```python
from build123d import *

# Parameters (mm, degrees)
SKETCH051_R             = 1.5
PAD022_DEPTH            = 3.5
SKETCH052_R             = 17.5
PAD003_DEPTH            = 12.5
SKETCH053_R             = 18.25
PAD004_DEPTH            = 4
SKETCH005_R             = 8
PAD023_DEPTH            = 2
SKETCH006_R             = 2.5
PAD021_DEPTH            = 12
BODY024_PLACEMENT_ANGLE = 90


with BuildPart() as part:
    # Sketch051 → Pad022 (new body)
    with BuildSketch(Plane.XY):
        with BuildLine():
            ThreePointArc((-16.780137, -7.175619), (0.077574, -18.249835), (16.840532, -7.032709))
            Line((23.588818, -4.651296), (16.840532, -7.032709))
            ThreePointArc((23.588818, -4.651296), (26.754582, -0.217457), (23.665308, 4.270011))
            Line((16.947438, 6.77103), (23.665308, 4.270011))
            ThreePointArc((16.947438, 6.77103), (0.049146, 18.249934), (-16.910725, 6.862207))
            Line((-16.910725, 6.862207), (-23.684267, 4.419805))
            ThreePointArc((-23.684267, 4.419805), (-26.870918, -0.10661), (-23.703302, -4.646365))
            Line((-23.703302, -4.646365), (-16.780137, -7.175619))
        make_face()
        with Locations((-22.015205, 0)):
            Circle(SKETCH051_R, mode=Mode.SUBTRACT)
        with Locations((21.805187, 0)):
            Circle(SKETCH051_R, mode=Mode.SUBTRACT)
    extrude(amount=PAD022_DEPTH)

    # Sketch052 (on Face11 of Pad022) → Pad003 (join)
    with BuildSketch(Plane(origin=(0, 0, 0), x_dir=(1, 0, 0), z_dir=(0, 0, -1))):
        Circle(SKETCH052_R)
    extrude(amount=PAD003_DEPTH)

    # Sketch053 (on Face14 of Pad003) → Pad004 (join)
    with BuildSketch(Plane(origin=(0, 0, -12.5), x_dir=(1, 0, 0), z_dir=(0, 0, -1))):
        Circle(SKETCH053_R)
    extrude(amount=PAD004_DEPTH)

    # Sketch005 (on Face16 of Pad004) → Pad023 (join)
    with BuildSketch(Plane.XY.offset(3.5)):
        Circle(SKETCH005_R)
    extrude(amount=PAD023_DEPTH)

    # Sketch006 (on Face18 of Pad023) → Pad021 (join)
    with BuildSketch(Plane.XY.offset(5.5)):
        Circle(SKETCH006_R)
    extrude(amount=PAD021_DEPTH)


with BuildPart() as part_1:
    # Body024 placement: moved
    add(part.part.moved(Location((0, 9.5, 80.3))).rotate(Axis((0, 9.5, 80.3), (-1, 0, 0)), BODY024_PLACEMENT_ANGLE))


solid = part_1.part
```
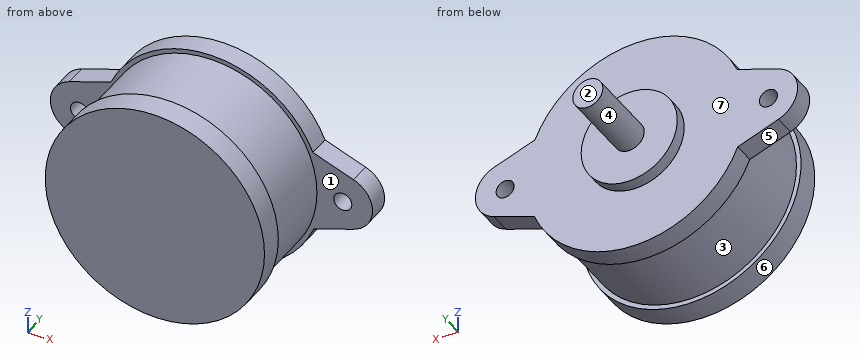
Geometry check sheet. Reference: the model listing, model coordinates, mm. Face numbers are marked on the shaded views. A direction names the side the tool comes from. Coordinates: 2 decimals unless noted, no trailing zeros. Loops run counter-clockwise (first coordinate to the right, second up) from the corner with the lowest first, then second, coordinate; pieces in that order, holes last.
Item 1: Sectioned sample at C-C, the plane y = 25.5. Record the boundary of the cut face in (x, z).
Item 2: Access from +Z, -Z, +X, -X, +Y, -Y to the whole of each face (thin tool, end or side, straight path). Record for the marked faces 5, 6 and 7.
Item 3: Release check for a two-part mould opening along Y. For the marked faces 1, 2, 3 and 4 record: released by +Y, released by -Y, zero draft, split by the parting line, or undercut.
Item 4: Sectioned sample at A-A, the plane z = 80.3. Record the boundary of the cut face in (x, y), then the cut area to 3 significant figures.
Item 5: Thickness scan on line 1 (X direction, y = 10.35, z = 80.3); line 2 (Y direction, x = 16, z = 87.5); line 3 (X direction, y = 10, z = 80). Record the ranges inside material, lowest first.
Item 6: Sectioned sample at D-D, the plane z = 89.5. Record the boundary of the cut face in (x, y), then the cut area to 3 significant figures.
Item 7: Go/stop test with flat-tipped pins: pin 1 Ø4 at (x, z) = (11.5, 81) entering from +Y; pin 2 Ø10 at (x, y) = (-13.5, 6) entering from -Z; pin 3 Ø11 at (x, z) = (9, 74.5) entering from +Y. Record where each tip stops, or that it passes through.
Item 8: Sectioned sample at B-B, the plane x = 0. Record the boundary of the cut face in (y, z).
Check result:
1. outline: circle Ø5 at (0, 80.3)
2. face 5: -Z, -X, +Y, -Y
2. face 6: -Y
2. face 7: +Y
3. face 1: undercut
3. face 2: released by +Y
3. face 3: undercut
3. face 4: zero draft
4. outline: (-26.87, 9.5) - (-23.52, 9.5) - (-23.52, 13) - (-26.87, 13) - close; (-20.52, 9.5) - (-17.5, 9.5) - (-17.5, -3) - (-18.25, -3) - (-18.25, -7) - (18.25, -7) - (18.25, -3) - (17.5, -3) - (17.5, 9.5) - (20.31, 9.5) - (20.31, 13) - (8, 13) - (8, 15) - (2.5, 15) - (2.5, 27) - (-2.5, 27) - (-2.5, 15) - (-8, 15) - (-8, 13) - (-20.52, 13) - close; (23.31, 9.5) - (26.75, 9.5) - (26.75, 13) - (23.31, 13) - close
4. area: 842 mm2
5. line 1: x = -26.87 to -23.52, -20.52 to 20.31, 23.31 to 26.75
5. line 2: y = -7 to -3, 9.5 to 13
5. line 3: x = -26.85 to -23.48, -20.55 to 20.34, 23.27 to 26.73
6. outline: (-15.76, -7) - (15.76, -7) - (15.76, -3) - (14.89, -3) - (14.89, 9.5) - (15.76, 9.5) - (15.76, 13) - (-15.76, 13) - (-15.76, 9.5) - (-14.89, 9.5) - (-14.89, -3) - (-15.76, -3) - close
6. area: 609 mm2
7. pin 1: stops at y = 13
7. pin 2: stops at z = 64.99
7. pin 3: stops at y = 15
8. outline: (-7, 62.05) - (-3, 62.05) - (-3, 62.8) - (9.5, 62.8) - (9.5, 62.05) - (13, 62.05) - (13, 72.3) - (15, 72.3) - (15, 77.8) - (27, 77.8) - (27, 82.8) - (15, 82.8) - (15, 88.3) - (13, 88.3) - (13, 98.55) - (9.5, 98.55) - (9.5, 97.8) - (-3, 97.8) - (-3, 98.55) - (-7, 98.55) - close
